The model under review builds one solid part; all positions refer to its coordinate system, in mm. Coordinates: 2 decimals unless noted, no trailing zeros. Loops run counter-clockwise (first coordinate to the right, second up) from the corner with the lowest first, then second, coordinate; pieces in that order, holes last. Notation, with made-up numbers: M 88,63 L 125,63 A33 cw 125,93 Z; hole C 68.25,51.5 d1. An arc over 180 degrees is marked long. Write item = value, one per line. Start each with the question number.
Q1. Clearance check with flat-ended pins moving along their axes: pin 1 Ø0.6 at (x, y) = (29.5, 1.5) entering from +Z; pin 2 Ø1 at (y, z) = (3, -138) entering from -X; pin 3 Ø3 at (y, z) = (2.5, -111) entering from +X. State where each tip first meets the part, or that it passes through.
Q2. We need section A-A on x = 10.5. Give the boundary of the cut face in (y, z).
Q3. Wall thickness on probe 1 along X at (y, z) = (5.1, -9.5); probe 2 along X at (y, z) = (5.2, -132.5); probe 3 along Z at (x, y) = (120, 2.85): over which ranges is each line inside the solid? List them lowest first.
Q4. We need section B-B on z = -99. Give the boundary of the cut face in (x, y).
from build123d import *

# Parameters (mm, degrees)
BOSS_EXTRUDE1_DEPTH = 5.5
FILLET1_R           = 2
FILLET2_R           = 3


with BuildPart() as part:
    # Sketch1 → Boss-Extrude1 (new body)
    with BuildSketch(Plane(origin=(0, 0, 0), x_dir=(1, 0, 0), z_dir=(0, 1, 0))):
        Polygon((0, 83.5), (0, 137), (30.5, 137), (30.5, 129.5), (29.3, 129.5), (29.3, 126.5), (30.5, 126.5), (30.5, 123), (33.5, 123), (33.5, 126.5), (34.7, 126.5), (34.7, 129.5), (33.5, 129.5), (33.5, 137), (53.5, 137), (53.5, 142.5), (83.5, 142.5), (83.5, 137), (137, 137), (137, 83.5), (155, 83.5), (155, 53.5), (137, 53.5), (137, 0), (83.5, 0), (83.5, -5.5), (53.5, -5.5), (53.5, 0), (33.5, 0), (33.5, 7.5), (34.7, 7.5), (34.7, 10.5), (33.5, 10.5), (33.5, 14), (30.5, 14), (30.5, 10.5), (29.3, 10.5), (29.3, 7.5), (30.5, 7.5), (30.5, 0), (0, 0), (0, 53.5), (-5.5, 53.5), (-5.5, 83.5), align=None)
    extrude(amount=BOSS_EXTRUDE1_DEPTH)

    # Fillet1
    fillet1_edges = [part.edges().sort_by_distance(p)[0] for p in [
        (-5.5, 2.75, -53.5),
        (-5.5, 2.75, -83.5),
        (53.5, 2.75, -142.5),
        (83.5, 2.75, -142.5),
        (83.5, 2.75, 5.5),
        (53.5, 2.75, 5.5),
    ]]
    fillet(fillet1_edges, radius=FILLET1_R)

    # Fillet2
    fillet2_edges = [part.edges().sort_by_distance(p)[0] for p in [
        (155, 2.75, -83.5),
        (155, 2.75, -53.5),
    ]]
    fillet(fillet2_edges, radius=FILLET2_R)


solid = part.part
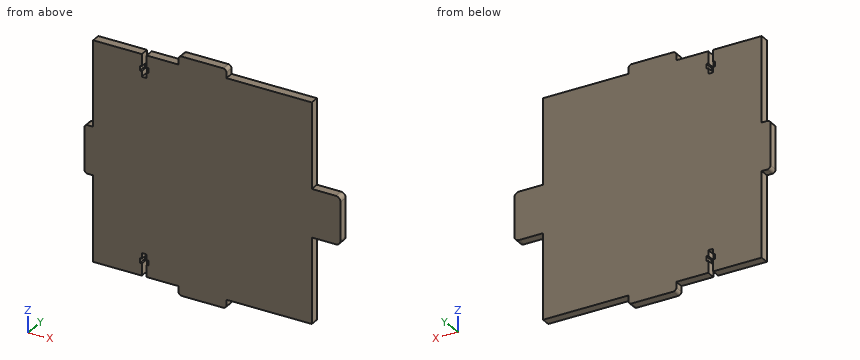
Returned:
q1.pin_1 = 0
q1.pin_2 = 53.5
q1.pin_3 = 137
q2.outline = M 0,-137 L 5.5,-137 L 5.5,0 L 0,0 Z
q3.probe_1 = 0 to 29.3, 34.7 to 137
q3.probe_2 = 0 to 30.5, 33.5 to 137
q3.probe_3 = -137 to 0
q4.outline = M 0,0 L 137,0 L 137,5.5 L 0,5.5 Z
